Could you check a few things on this model? Use its own coordinates, in mm. A direction names the side the tool comes from. Give positions to 0.01 mm unless a question says otherwise; leave off trailing zeros. Loops run counter-clockwise (first coordinate to the right, second up) from the corner with the lowest first, then second, coordinate; pieces in that order, holes last. Notation, with made-up numbers: (61, 18) - (65, 18) arc R25 ccw to (65, 50) - close; hole circle Ø5 at (82.5, 76). An arc over 180 degrees is marked (long way). Use CSV: the item, a comma, the result in double quotes.
from build123d import *

# Parameters (mm, degrees)
SKETCH_1_W             = 42
SKETCH_1_H             = 42
EXTRUDE_1_DEPTH        = 39
FILLET_1_R             = 10
HOLE_WIZARD_M3_1_D     = 2.5
HOLE_WIZARD_M3_1_DEPTH = 7.5
HOLE_WIZARD_M3_1_TIP   = 0.751075774
SKETCH_4_R             = 11
EXTRUDE_2_DEPTH        = 2
SKETCH_5_R             = 2.5
EXTRUDE_3_DEPTH        = 23


with BuildPart() as part:
    # 草图1 → 凸台-拉伸1 (new body)
    with BuildSketch(Plane.XY):
        with Locations((21, 21)):
            Rectangle(SKETCH_1_W, SKETCH_1_H)
    extrude(amount=EXTRUDE_1_DEPTH)

    # 圆角1
    fillet_1_edges = [part.edges().sort_by_distance(p)[0] for p in [
        (0, 42, 19.5),
        (42, 42, 19.5),
        (42, 0, 19.5),
        (0, 0, 19.5),
    ]]
    fillet(fillet_1_edges, radius=FILLET_1_R)

    # M3 螺纹孔1
    with Locations(Plane.XY.offset(39)):
        with Locations((5.5, 36.5), (36.5, 36.5), (36.5, 5.5), (5.5, 5.5)):
            Hole(HOLE_WIZARD_M3_1_D / 2, depth=HOLE_WIZARD_M3_1_DEPTH)
            with Locations((0, 0, -(HOLE_WIZARD_M3_1_DEPTH + HOLE_WIZARD_M3_1_TIP / 2))):  # 118° drill point
                Cone(0, HOLE_WIZARD_M3_1_D / 2, HOLE_WIZARD_M3_1_TIP, mode=Mode.SUBTRACT)

    # 草图4 → 凸台-拉伸2 (add)
    with BuildSketch(Plane.XY.offset(39)):
        with Locations((21, 21)):
            Circle(SKETCH_4_R)
    extrude(amount=EXTRUDE_2_DEPTH)

    # 草图5 → 凸台-拉伸3 (add)
    with BuildSketch(Plane.XY.offset(41)):
        with Locations((21, 21)):
            Circle(SKETCH_5_R)
    extrude(amount=EXTRUDE_3_DEPTH)


solid = part.part
1) I need wall thicknesses on line 1 along X through (y, z) = (5, 35); line 2 along X through (y, z) = (35.5, 36.5); line 3 along Y through (x, z) = (36.5, 33.75). Which ranges of each line are inside material? Lowest first, please.
Answer below:
line 1,"x = 1.34 to 4.35, 6.65 to 35.35, 37.65 to 40.66"
line 2,"x = 0.63 to 4.75, 6.25 to 35.75, 37.25 to 41.37"
line 3,"y = 1.07 to 4.25, 6.75 to 35.25, 37.75 to 40.93"
2) I'm going to push flat-ended pins straight in: P1, Ø1, axis at x = 14, y = 27, coming from the -Z side; P2, Ø3, axis at x = 5.5, y = 5.5, coming from the +Z side; P3, Ø12.5, axis at x = 12, y = 12, coming from the +Z side. Where does each tip first touch, or does it pass through?
Answer below:
P1,"stops at z = 0"
P2,"stops at z = 39"
P3,"stops at z = 41"
3) Which directions (+Z, -Z, +X, -X, +Y, -Y) give clear straight access to the entire face, cutting with the end or side of a thin tool? Please do faces 5 (the flat face through (21, 0, 19)), 6 (the cylindrical face through (19.16, 22.69, 52.34)).
Answer below:
face 5,"+Z, -Z, +X, -X, -Y"
face 6,"+Z"
4) Suppose I cut it at A-A (x = 21). Please give me the cut outline in (y, z), plus the area to 3 significant figures.
Answer below:
outline,"(0, 0) - (42, 0) - (42, 39) - (32, 39) - (32, 41) - (23.5, 41) - (23.5, 64) - (18.5, 64) - (18.5, 41) - (10, 41) - (10, 39) - (0, 39) - close"
area,"1,800 mm2"
5) We'd pull the mould along Y, two halves only. Please class faces 1 (the conical face through (36.71, 5.57, 30.88)), 2 (the cylindrical face through (37.49, 35.74, 35.2)), 3 (the flat face through (21, 24, 41)), 4 (the cylindrical face through (2.85, 38.99, 19.77)): +Y half, -Y half, draft (parallel to the pull), parting line (faces both ways), or undercut.
Answer below:
face 1,"undercut"
face 2,"undercut"
face 3,"draft"
face 4,"+Y half"
6) Suppose I cut it at D-D (x = 29). Please give me the cut outline in (y, z), plus the area to 3 significant figures.
Answer below:
outline,"(0, 0) - (42, 0) - (42, 39) - (28.55, 39) - (28.55, 41) - (13.45, 41) - (13.45, 39) - (0, 39) - close"
area,"1,670 mm2"
7) Suppose I cut it at C-C (z = 28.5). Please give me the cut outline in (x, y).
Answer below:
outline,"(0, 10) arc R10 ccw to (10, 0) - (32, 0) arc R10 ccw to (42, 10) - (42, 32) arc R10 ccw to (32, 42) - (10, 42) arc R10 ccw to (0, 32) - close"
